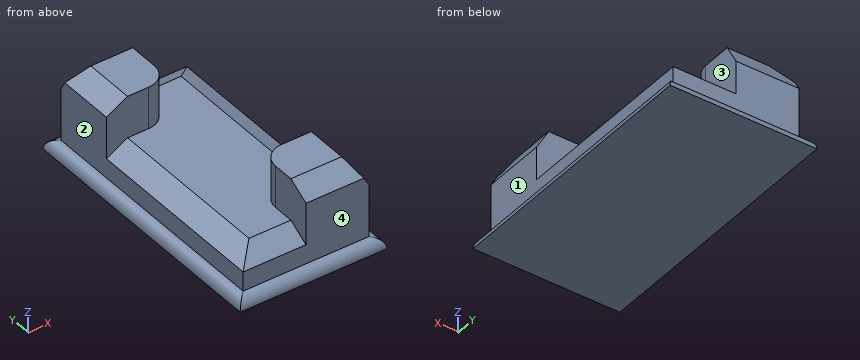
from build123d import *

# Parameters (mm, degrees)
F1_DEPTH    = 6.35
F2_DEPTH    = 25.4
F3_DEPTH    = 50.8
F4_C1_SIZE2 = 12.7
F4_C1_SIZE  = 7.3323484187
F4_C2_SIZE2 = 12.7
F4_C2_SIZE  = 7.3323484187
F4_C3_SIZE2 = 7.3323484187
F4_C3_SIZE  = 12.7
F4_C4_SIZE2 = 12.7
F4_C4_SIZE  = 7.3323484187
F4_C5_SIZE2 = 12.7
F4_C5_SIZE  = 7.3323484187
F4_C6_SIZE2 = 12.7
F4_C6_SIZE  = 7.3323484187
F4_C7_SIZE2 = 12.7
F4_C7_SIZE  = 7.3323484187
F4_C8_SIZE2 = 12.7
F4_C8_SIZE  = 7.3323484187
F5_R        = 6.34999


# Not quite as in the source:
# - a fillet or chamfer is up to 0.001 mm smaller than in the source, because OpenCascade refuses the exact size


with BuildPart() as f1:
    # F0 (on Top) → F1 (new body)
    with BuildSketch(Plane.XY):
        Polygon((-38.1, 38.1), (-38.1, 76.2), (0, 76.2), (38.1, 76.2), (38.1, 82.55), (-44.45, 82.55), (-44.45, -82.55), (-38.1, -82.55), (-38.1, -76.2), align=None)
        Polygon((38.1, 82.55), (38.1, 76.2), (38.1, -38.1), (38.1, -76.2), (0, -76.2), (-38.1, -76.2), (-38.1, -82.55), (44.45, -82.55), (44.45, 82.55), align=None)
    extrude(amount=F1_DEPTH)

    # F0 (on Top) → F2 (join)
    with BuildSketch(Plane.XY):
        with BuildLine():
            Line((38.1, 76.2), (0, 76.2))
            Line((0, 76.2), (0, 50.8))
            ThreePointArc((0, 50.8), (-3.7197438789, 41.8197438789), (-12.7, 38.1))
            Line((-12.7, 38.1), (-38.1, 38.1))
            Line((-38.1, 38.1), (-38.1, -76.2))
            Line((-38.1, -76.2), (0, -76.2))
            Line((0, -76.2), (0, -50.8))
            ThreePointArc((0, -50.8), (3.7197438789, -41.8197438789), (12.7, -38.1))
            Line((12.7, -38.1), (38.1, -38.1))
            Line((38.1, -38.1), (38.1, 76.2))
        make_face()
    extrude(amount=F2_DEPTH)

    # F0 (on Top) → F3 (join)
    with BuildSketch(Plane.XY):
        with BuildLine():
            Line((0, 76.2), (-38.1, 76.2))
            Line((-38.1, 76.2), (-38.1, 38.1))
            Line((-38.1, 38.1), (-12.7, 38.1))
            ThreePointArc((-12.7, 38.1), (-3.7197438789, 41.8197438789), (0, 50.8))
            Line((0, 50.8), (0, 76.2))
        make_face()
        with BuildLine():
            Line((38.1, -76.2), (38.1, -38.1))
            Line((38.1, -38.1), (12.7, -38.1))
            ThreePointArc((12.7, -38.1), (3.7197438789, -41.8197438789), (0, -50.8))
            Line((0, -50.8), (0, -76.2))
            Line((0, -76.2), (38.1, -76.2))
        make_face()
    extrude(amount=F3_DEPTH)

    # F4: chamfer of 12.7 x 7.3323484187 on 8 edges, made by hand

    # F4_c1
    f4_c1_edges = [f1.edges().sort_by_distance(p)[0] for p in [
        (-19.05, -76.2, 25.4),
    ]]
    f4_c1_side = f1.faces().sort_by_distance((-19.05, -76.2, 25.2533530316))[0]
    chamfer(f4_c1_edges, length=F4_C1_SIZE, length2=F4_C1_SIZE2, reference=f4_c1_side)

    # F4_c2
    f4_c2_edges = [f1.edges().sort_by_distance(p)[0] for p in [
        (19.05, -76.2, 50.8),
    ]]
    f4_c2_side = f1.faces().sort_by_distance((19.05, -76.2, 50.6533530316))[0]
    chamfer(f4_c2_edges, length=F4_C2_SIZE, length2=F4_C2_SIZE2, reference=f4_c2_side)

    # F4_c3
    f4_c3_edges = [f1.edges().sort_by_distance(p)[0] for p in [
        (38.1, -50.8, 50.8),
    ]]
    f4_c3_side = f1.faces().sort_by_distance((38.1, -50.8, 50.6533530316))[0]
    chamfer(f4_c3_edges, length=F4_C3_SIZE, length2=F4_C3_SIZE2, reference=f4_c3_side)

    # F4_c4
    f4_c4_edges = [f1.edges().sort_by_distance(p)[0] for p in [
        (38.1, 19.05, 25.4),
    ]]
    f4_c4_side = f1.faces().sort_by_distance((38.1, 19.05, 25.2533530316))[0]
    chamfer(f4_c4_edges, length=F4_C4_SIZE, length2=F4_C4_SIZE2, reference=f4_c4_side)

    # F4_c5
    f4_c5_edges = [f1.edges().sort_by_distance(p)[0] for p in [
        (12.7, 76.2, 25.4),
    ]]
    f4_c5_side = f1.faces().sort_by_distance((12.7, 76.2, 25.2533530316))[0]
    chamfer(f4_c5_edges, length=F4_C5_SIZE, length2=F4_C5_SIZE2, reference=f4_c5_side)

    # F4_c6
    f4_c6_edges = [f1.edges().sort_by_distance(p)[0] for p in [
        (-38.1, -12.7, 25.4),
    ]]
    f4_c6_side = f1.faces().sort_by_distance((-38.1, -12.7, 25.2533530316))[0]
    chamfer(f4_c6_edges, length=F4_C6_SIZE, length2=F4_C6_SIZE2, reference=f4_c6_side)

    # F4_c7
    f4_c7_edges = [f1.edges().sort_by_distance(p)[0] for p in [
        (-19.05, 76.2, 50.8),
    ]]
    f4_c7_side = f1.faces().sort_by_distance((-19.05, 76.0533530316, 50.8))[0]
    chamfer(f4_c7_edges, length=F4_C7_SIZE, length2=F4_C7_SIZE2, reference=f4_c7_side)

    # F4_c8
    f4_c8_edges = [f1.edges().sort_by_distance(p)[0] for p in [
        (-38.1, 53.4838257906, 50.8),
    ]]
    f4_c8_side = f1.faces().sort_by_distance((-38.1, 53.4838257906, 50.6533530316))[0]
    chamfer(f4_c8_edges, length=F4_C8_SIZE, length2=F4_C8_SIZE2, reference=f4_c8_side)

    # F5 (radius 6.35 in the source; OpenCascade refuses exactly that, so slightly less here)
    f5_edges = [f1.edges().sort_by_distance(p)[0] for p in [
        (-44.45, 0, 6.35),
        (0, 82.55, 6.35),
        (44.45, 0, 6.35),
        (0, -82.55, 6.35),
    ]]
    fillet(f5_edges, radius=F5_R)


solid = f1.part
Can you work these out from the model? Positions are in its coordinate system, mm. Face numbers are marked on the shaded views. A direction names the side the tool comes from. Coordinates: 2 decimals unless noted, no trailing zeros. Order: outer loops, then holes, each group sorted by start corner. A loop starts at its lowest first (then second) coordinate and runs counter-clockwise, first axis right, second up. Notation, with made-up numbers: M 68.5,-23.75 L 75.5,-23.75 A18 ccw 75.5,-7.75 Z; hole C 29.25,23.25 d3. An arc over 180 degrees is marked long. Write item = value, one per line.
(1) Suppose I cut it at D-D on z = 13.5. Please give me the cut outline in (x, y), plus the area to 3 significant figures.
Results are:
outline = M -38.1,-76.2 L 38.1,-76.2 L 38.1,76.2 L -38.1,76.2 Z
area = 11,600 mm2
(2) For pin 1 Ø12.5 at (x, z) = (30, 34) entering from +Y; pin 2 Ø10 at (x, z) = (-34.5, 9.5) entering from +Y; pin 3 Ø12 at (y, z) = (-64.5, 21) entering from +X, each with a flat end and sliding along its axis, tell me the tip position at first contact or that it passes through.
Results are:
pin_1 = -38.1
pin_2 = 80.68
pin_3 = 38.1
(3) I need wall thicknesses on line 1 along Z through (x, y) = (-7, -30); line 2 along Y through (x, z) = (18, 10.5); line 3 along Y through (x, z) = (-18, 26.5). Which ranges of each line are inside material? Lowest first, please. Write a range as [from, to].
Results are:
line_1 = [0, 25.4]
line_2 = [-76.2, 76.2]
line_3 = [38.1, 76.2]
(4) For the marked faces 1, 2, 3 and 4, which set-ups out of +Z, -Z, +X, -X, +Y, -Y let a thin tool reach every point of the face, with its end or its side?
Results are:
face_1 = +Z, +X, +Y, -Y
face_2 = +Z, -X, +Y, -Y
face_3 = +Z, +X, +Y
face_4 = +Z, +X, -X, -Y
(5) Suppose I cut it at A-A on z = 34.5. Please give me the cut outline in (x, y).
Results are:
outline = M -38.1,38.1 L -12.7,38.1 A12.7 ccw 0,50.8 L 0,76.2 L -38.1,76.2 Z; M 0,-76.2 L 38.1,-76.2 L 38.1,-38.1 L 12.7,-38.1 A12.7 ccw 0,-50.8 Z
